Design review of the part shown in the three views and the two pictorial views. Dimensions are in mm from the part's minimum x, y and z. Round coordinates to 2 decimals unless told otherwise and drop trailing zeros. Loops run counter-clockwise (first coordinate to the right, second up) from the corner with the lowest first, then second, coordinate; pieces in that order, holes last. Notation, with made-up numbers: (-40, -25.5) -> (8, -25.5) arc R16 cw to (8, -11.5) -> close; hole circle Ø10 at (14.25, -27.75). An arc over 180 degrees is marked (long way). One line per question, with ' | ' between items. Start each with the question number.
1. Consider section C-C (y = 3.75). Write out the cut boundary in (x, z) (1 decimal), and give its area (3 significant figures).
2. Consider section D-D (z = 133.5). Write out the cut boundary in (x, y) (1 decimal), and give its area (3 significant figures).
3. Consider section B-B (x = 77.5). Write out the cut boundary in (y, z).
4. Draft analysis for pull direction Y (two halves, no side actions). For the marked faces 1 and 2, state which applies: pulls with the +Y half, pulls with the -Y half, needs draft (parallel to the pull), parting line crosses it, or undercut.
5. Wall thickness on line 1 along X through (y, z) = (3.2, 77.5); line 2 along Z through (x, y) = (87, 1.55) (1 decimal): over which ranges is each line inside the solid? List them lowest first.
6. Consider section A-A (z = 77.5). Write out the cut boundary in (x, y), and give its area (3 significant figures).
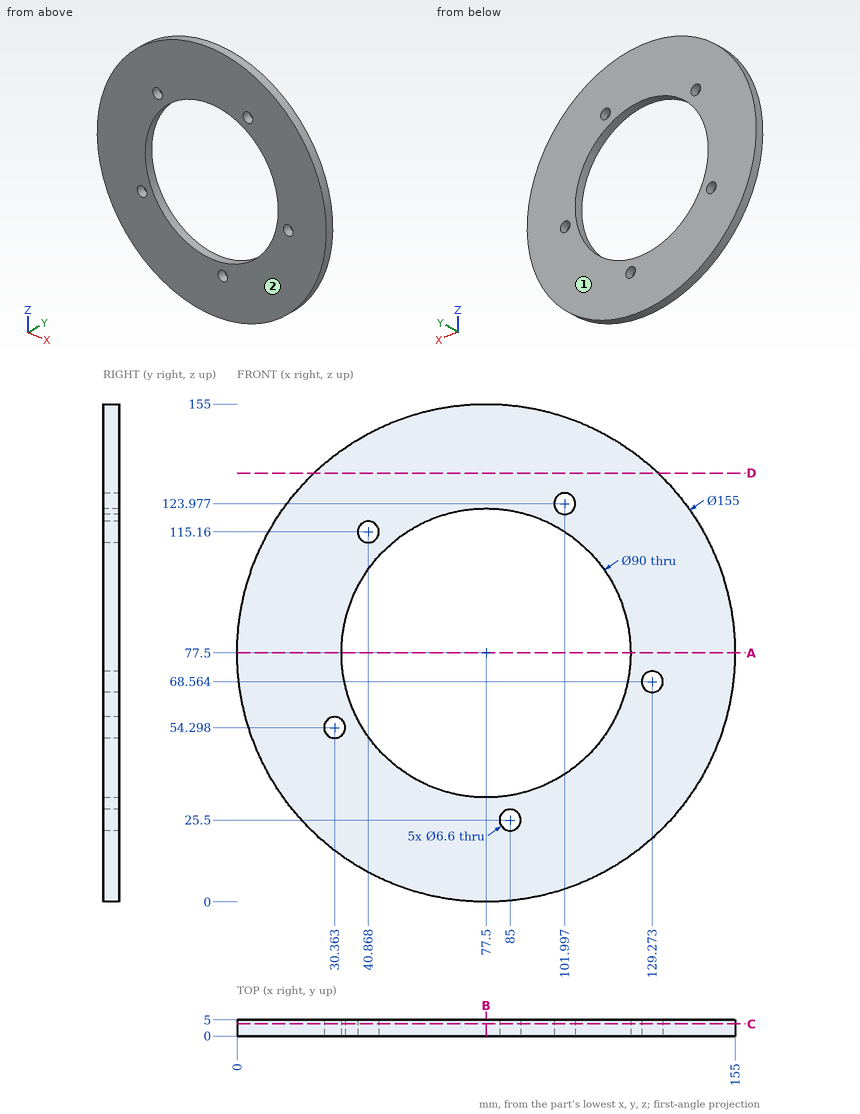
Answer block:
1) outline: circle Ø155 at (77.5, 77.5); hole circle Ø6.6 at (30.4, 54.3); hole circle Ø90 at (77.5, 77.5); hole circle Ø6.6 at (40.9, 115.2); hole circle Ø6.6 at (85, 25.5); hole circle Ø6.6 at (102, 124); hole circle Ø6.6 at (129.3, 68.6) | area: 12,300 mm2
2) outline: (23.9, 0) -> (131.1, 0) -> (131.1, 5) -> (23.9, 5) -> close | area: 536 mm2
3) outline: (0, 0) -> (5, 0) -> (5, 32.5) -> (0, 32.5) -> close; (0, 122.5) -> (5, 122.5) -> (5, 155) -> (0, 155) -> close
4) face 1: pulls with the +Y half | face 2: pulls with the -Y half
5) line 1: x = 0 to 32.5, 122.5 to 155 | line 2: z = 0.6 to 22.9, 28.1 to 33.5, 121.5 to 154.4
6) outline: (0, 0) -> (32.5, 0) -> (32.5, 5) -> (0, 5) -> close; (122.5, 0) -> (155, 0) -> (155, 5) -> (122.5, 5) -> close | area: 325 mm2
